CAD build for the part. Positions are in the model's coordinates, mm. Face numbers are marked on the shaded views. A direction names the side the tool comes from. Coordinates: 2 decimals unless noted, no trailing zeros. Write each loop counter-clockwise with the first axis right and the second up, starting at its lowest first coordinate (ties: lowest second). Pieces come first, ordered by that corner, then holes. Notation, with made-up numbers: (49.5, -2.75) - (59.5, -2.75) arc R23 ccw to (59.5, 30.25) - close; hole circle Ø11 at (20.5, 50). An arc over 180 degrees is marked (long way). Answer in a Markdown table with one row per item. Add a question column.
Q1. Band-saw the part on A-A (z = 28.5). List the corners of the cut face in (x, y).
Q2. Drill centre lines: line 1 along X through (y, z) = (-24, 7); line 2 along X through (y, z) = (-14, 20); line 3 along Z through (x, y) = (-16, 27). Where is each one in solid material? Low to high. Write a range as from..to.
Q3. Band-saw the part on C-C (x = -31.5). List the corners of the cut face in (y, z), and give its area (3 significant figures).
Q4. Band-saw the part on B-B (y = -18). List the corners of the cut face in (x, z).
Q5. Two-plate mould, pull along X, no slides. Class the marked faces 4, 5 and 6: +X half, -X half, draft (parallel to the pull), parting line (faces both ways), or undercut.
Q6. Pin check, flat tips, straight feed: pin 1 (4 mm diameter, centred on y = 12, z = 5.5, fed in from -X); pin 2 (10 mm diameter, centred on y = -17, z = 10, fed in from -X); pin 3 (1.5 mm diameter, centred on x = 15, y = 28.5, fed in from -Z). Stop position of each tip, or through.
Q7. 3-axis set-ups, long thin cutter, end or side, ignore diameter. For the marked faces 1, 2 and 3: which of +Z, -Z, +X, -X, +Y, -Y reach the whole face in a straight line?
```python
from build123d import *

# Parameters (mm, degrees)
F1_DEPTH     = 30
F3_DEPTH     = 30
F4_DEPTH     = 25
F5_T1_DEPTH  = 97.9548533656
F5_T3_DEPTH  = 20
F5_T5_DEPTH  = 20.7033743208
F5_T7_DEPTH  = 97.9794901198
F5_T9_DEPTH  = 20
F5_T12_ANGLE = 75.8911885194
F5_T14_ANGLE = 104.1088114806
F5_T16_ANGLE = 75.2928746344
F5_T20_DEPTH = 43.6443917162
F5_T23_ANGLE = 75.8339831116
F5_T25_ANGLE = 104.1660168884
F5_T27_ANGLE = 78.1908320725
F5_T31_DEPTH = 42.9024259572
F5_T37_DEPTH = 42.9024259572
F5_T41_DEPTH = 43.6443917162


# Not quite as in the source:
# - a fillet or chamfer that OpenCascade refuses, or shapes differently, is made with other operations: its cross-section is extruded or revolved along the edge and cut away or added
# - the program builds the solid bodies; features that only make, move or delete a surface that nothing else refers to are left out


with BuildPart() as f1:
    # F0 (on Top) → F1 (new body)
    with BuildSketch(Plane.XY):
        with BuildLine():
            Line((9.3227045948, 64.7266464915), (-11.3806697261, 64.7266464915))
            ThreePointArc((-11.3806697261, 64.7266464915), (-15.9925167381, 63.1411090315), (-18.6544287642, 59.0548777281))
            Line((-18.6544287642, 59.0548777281), (-42.5323117917, -35.9451222719))
            ThreePointArc((-42.5323117917, -35.9451222719), (-41.1730152936, -42.3852005206), (-35.2585527536, -45.2733535085))
            Line((-35.2585527536, -45.2733535085), (-15.2585527536, -45.2733535085))
            ThreePointArc((-15.2585527536, -45.2733535085), (-10.6776494918, -43.7118150354), (-8.004281346, -39.6774402567))
            Line((-8.004281346, -39.6774402567), (-0.1883919579, -9.9001294455))
            Line((-0.1883919579, -9.9001294455), (5.9601953638, -39.3082485958))
            ThreePointArc((5.9601953638, -39.3082485958), (8.571852392, -43.5940799733), (13.3014552741, -45.2733535085))
            Line((13.3014552741, -45.2733535085), (33.3014552741, -45.2733535085))
            ThreePointArc((33.3014552741, -45.2733535085), (39.2182193635, -42.3822473792), (40.5733853395, -35.9378608981))
            Line((40.5733853395, -35.9378608981), (16.5946346602, 59.0621391019))
            ThreePointArc((16.5946346602, 59.0621391019), (13.9315984654, 63.1434105808), (9.3227045948, 64.7266464915))
        make_face()
        with BuildLine():
            ThreePointArc((9.3227045948, 59.7266464915), (10.8590025517, 59.1989011879), (11.7466812833, 57.8384773616))
            Line((11.7466812833, 57.8384773616), (35.7254319626, -37.1615226384))
            ThreePointArc((35.7254319626, -37.1615226384), (35.2737099706, -39.3096514654), (33.3014552741, -40.2733535085))
            Line((33.3014552741, -40.2733535085), (13.3014552741, -40.2733535085))
            ThreePointArc((13.3014552741, -40.2733535085), (11.72492098, -39.7135956635), (10.8543686373, -38.2849852043))
            Line((10.8543686373, -38.2849852043), (3.2176150905, -1.7591059289))
            ThreePointArc((3.2176150905, -1.7591059289), (2.3470627478, -0.3304954698), (0.7705284538, 0.2292623753))
            Line((0.7705284538, 0.2292623753), (-0.7705284538, 0.2292623753))
            ThreePointArc((-0.7705284538, 0.2292623753), (-2.2974962077, -0.2912504491), (-3.188618923, -1.6360420419))
            Line((-3.188618923, -1.6360420419), (-12.8404622844, -38.4080490913))
            ThreePointArc((-12.8404622844, -38.4080490913), (-13.7315849996, -39.7528406842), (-15.2585527536, -40.2733535085))
            Line((-15.2585527536, -40.2733535085), (-35.2585527536, -40.2733535085))
            ThreePointArc((-35.2585527536, -40.2733535085), (-37.2300402669, -39.3106358459), (-37.6831390996, -37.1639430963))
            Line((-37.6831390996, -37.1639430963), (-13.8052560721, 57.8360569037))
            ThreePointArc((-13.8052560721, 57.8360569037), (-12.9179520634, 59.1981340048), (-11.3806697261, 59.7266464915))
            Line((-11.3806697261, 59.7266464915), (9.3227045948, 59.7266464915))
        make_face(mode=Mode.SUBTRACT)
    extrude(amount=F1_DEPTH)

    # F0 (on Top) → F3 (join)
    with BuildSketch(Plane.XY):
        with BuildLine():
            Line((35.7254319626, -37.1615226384), (11.7466812833, 57.8384773616))
            ThreePointArc((11.7466812833, 57.8384773616), (10.8590025517, 59.1989011879), (9.3227045948, 59.7266464915))
            Line((9.3227045948, 59.7266464915), (-11.3806697261, 59.7266464915))
            ThreePointArc((-11.3806697261, 59.7266464915), (-12.9179520634, 59.1981340048), (-13.8052560721, 57.8360569037))
            Line((-13.8052560721, 57.8360569037), (-37.6831390996, -37.1639430963))
            ThreePointArc((-37.6831390996, -37.1639430963), (-37.2300402669, -39.3106358459), (-35.2585527536, -40.2733535085))
            Line((-35.2585527536, -40.2733535085), (-15.2585527536, -40.2733535085))
            ThreePointArc((-15.2585527536, -40.2733535085), (-13.7315849996, -39.7528406842), (-12.8404622844, -38.4080490913))
            Line((-12.8404622844, -38.4080490913), (-3.188618923, -1.6360420419))
            ThreePointArc((-3.188618923, -1.6360420419), (-2.2974962077, -0.2912504491), (-0.7705284538, 0.2292623753))
            Line((-0.7705284538, 0.2292623753), (0.7705284538, 0.2292623753))
            ThreePointArc((0.7705284538, 0.2292623753), (2.3470627478, -0.3304954698), (3.2176150905, -1.7591059289))
            Line((3.2176150905, -1.7591059289), (10.8543686373, -38.2849852043))
            ThreePointArc((10.8543686373, -38.2849852043), (11.72492098, -39.7135956635), (13.3014552741, -40.2733535085))
            Line((13.3014552741, -40.2733535085), (33.3014552741, -40.2733535085))
            ThreePointArc((33.3014552741, -40.2733535085), (35.2737099706, -39.3096514654), (35.7254319626, -37.1615226384))
        make_face()
        Polygon((2.9763113208, 15.0989185788), (-2.9763113208, 15.0989185788), (-0.655874512, 25.3615314645), (0.655874512, 25.3615314645), align=None, mode=Mode.SUBTRACT)
    extrude(amount=F3_DEPTH)

    # F0 (on Top) → F4 (cut)
    with BuildSketch(Plane.XY):
        with BuildLine():
            Line((35.7254319626, -37.1615226384), (11.7466812833, 57.8384773616))
            ThreePointArc((11.7466812833, 57.8384773616), (10.8590025517, 59.1989011879), (9.3227045948, 59.7266464915))
            Line((9.3227045948, 59.7266464915), (-11.3806697261, 59.7266464915))
            ThreePointArc((-11.3806697261, 59.7266464915), (-12.9179520634, 59.1981340048), (-13.8052560721, 57.8360569037))
            Line((-13.8052560721, 57.8360569037), (-37.6831390996, -37.1639430963))
            ThreePointArc((-37.6831390996, -37.1639430963), (-37.2300402669, -39.3106358459), (-35.2585527536, -40.2733535085))
            Line((-35.2585527536, -40.2733535085), (-15.2585527536, -40.2733535085))
            ThreePointArc((-15.2585527536, -40.2733535085), (-13.7315849996, -39.7528406842), (-12.8404622844, -38.4080490913))
            Line((-12.8404622844, -38.4080490913), (-3.188618923, -1.6360420419))
            ThreePointArc((-3.188618923, -1.6360420419), (-2.2974962077, -0.2912504491), (-0.7705284538, 0.2292623753))
            Line((-0.7705284538, 0.2292623753), (0.7705284538, 0.2292623753))
            ThreePointArc((0.7705284538, 0.2292623753), (2.3470627478, -0.3304954698), (3.2176150905, -1.7591059289))
            Line((3.2176150905, -1.7591059289), (10.8543686373, -38.2849852043))
            ThreePointArc((10.8543686373, -38.2849852043), (11.72492098, -39.7135956635), (13.3014552741, -40.2733535085))
            Line((13.3014552741, -40.2733535085), (33.3014552741, -40.2733535085))
            ThreePointArc((33.3014552741, -40.2733535085), (35.2737099706, -39.3096514654), (35.7254319626, -37.1615226384))
        make_face()
        Polygon((2.9763113208, 15.0989185788), (-2.9763113208, 15.0989185788), (-0.655874512, 25.3615314645), (0.655874512, 25.3615314645), align=None, mode=Mode.SUBTRACT)
    extrude(amount=F4_DEPTH, mode=Mode.SUBTRACT)

    # F5: chamfer of 5 on 1 edges, made by hand

    # F5_s2 → F5_t1 (cut)
    with BuildSketch(Plane(origin=(12.8527529512, 51.135669312, 0), x_dir=(0, 0, 1), z_dir=(-0.2437641649, -0.9698345384, 0))):
        Polygon((0, 27.4871722621), (5, 32.4871722621), (0, 32.4871722621), align=None)
    extrude(amount=F5_T1_DEPTH, mode=Mode.SUBTRACT)

    # F5_s4 → F5_t3 (cut)
    with BuildSketch(Plane.YZ.offset(-35.2585527536)):
        Polygon((-40.2733535085, 0), (-45.2733535085, 5), (-45.2733535085, 0), align=None)
    extrude(amount=F5_T3_DEPTH, mode=Mode.SUBTRACT)

    # F5_s6 → F5_t5 (cut)
    with BuildSketch(Plane.YZ.offset(-11.3806697261)):
        Polygon((64.7266464915, 5), (59.7266464915, 0), (64.7266464915, 0), align=None)
    extrude(amount=F5_T5_DEPTH, mode=Mode.SUBTRACT)

    # F5_s8 → F5_t7 (cut)
    with BuildSketch(Plane(origin=(10.9578014799, -43.4130682832, 0), x_dir=(0, 0, 1), z_dir=(-0.2447323481, 0.9695906754, 0))):
        Polygon((5, 30.5444190123), (0, 25.5444190123), (0, 30.5444190123), align=None)
    extrude(amount=F5_T7_DEPTH, mode=Mode.SUBTRACT)

    # F5_s10 → F5_t9 (cut)
    with BuildSketch(Plane.YZ.offset(13.3014552741)):
        Polygon((-40.2733535085, 0), (-45.2733535085, 5), (-45.2733535085, 0), align=None)
    extrude(amount=F5_T9_DEPTH, mode=Mode.SUBTRACT)

    # F5_s11 → F5_t12 (revolve, cut)
    with BuildSketch(Plane.YZ.offset(-11.3806697261)):
        Polygon((59.7266464915, 0), (64.7266464915, 5), (64.7266464915, 0), align=None)
    revolve(axis=Axis((-11.3806697261, 57.2266464915, 0), (0, 0, 1)), revolution_arc=F5_T12_ANGLE, mode=Mode.SUBTRACT)

    # F5_s13 → F5_t14 (revolve, cut)
    with BuildSketch(Plane(origin=(-11.0251300763, -43.864330688, 0), x_dir=(0, 0, 1), z_dir=(0.2437641649, 0.9698345384, 0))):
        Polygon((0, -27.4871722621), (5, -32.4871722621), (0, -32.4871722621), align=None)
    revolve(axis=Axis((-35.2585527536, -37.7733535085, 0), (0, 0, 1)), revolution_arc=F5_T14_ANGLE, mode=Mode.SUBTRACT)

    # F5_s15 → F5_t16 (revolve, cut)
    with BuildSketch(Plane.YZ.offset(-15.2585527536)):
        Polygon((-40.2733535085, 0), (-45.2733535085, 5), (-45.2733535085, 0), align=None)
    revolve(axis=Axis((-15.2585527536, -37.7733535085, 0), (0, 0, 1)), revolution_arc=F5_T16_ANGLE, mode=Mode.SUBTRACT)


with BuildPart() as f5_tool18:
    # F5_s19 → F5_t20 (new body)
    with BuildSketch(Plane(origin=(-10.2591099413, -39.0855973263, 0), x_dir=(0, 0, 1), z_dir=(0.2538782331, 0.9672361877, 0))):
        Polygon((0, -2.6687921481), (5, 2.3312078519), (0, 2.3312078519), align=None)
    extrude(amount=F5_T20_DEPTH)

    split(bisect_by=Plane(origin=(-2.1637067448, -0.4523832276, 0), x_dir=(0, 0, 1), z_dir=(-0.9788346547, -0.2046526783, 0)), keep=Keep.TOP)


with BuildPart() as f1_1:
    add(f1.part)

    # F5_t17: cut F5_tool18
    add(f5_tool18.part, mode=Mode.SUBTRACT)

    # F5_s22 → F5_t23 (revolve, cut)
    with BuildSketch(Plane(origin=(-13.0209491994, 51.5869317168, 0), x_dir=(0, 0, 1), z_dir=(0.2447323481, -0.9695906754, 0))):
        Polygon((5, -30.5444190123), (0, -25.5444190123), (0, -30.5444190123), align=None)
    revolve(axis=Axis((9.3227045948, 57.2266464915, 0), (0, 0, 1)), revolution_arc=F5_T23_ANGLE, mode=Mode.SUBTRACT)

    # F5_s24 → F5_t25 (revolve, cut)
    with BuildSketch(Plane.YZ.offset(33.3014552741)):
        Polygon((-40.2733535085, 0), (-45.2733535085, 5), (-45.2733535085, 0), align=None)
    revolve(axis=Axis((33.3014552741, -37.7733535085, 0), (0, 0, 1)), revolution_arc=F5_T25_ANGLE, mode=Mode.SUBTRACT)

    # F5_s26 → F5_t27 (revolve, cut)
    with BuildSketch(Plane(origin=(8.1239021086, -38.8558653682, 0), x_dir=(0, 0, 1), z_dir=(-0.2046526783, 0.9788346547, 0))):
        Polygon((0, 2.7895074164), (5, -2.2104925836), (0, -2.2104925836), align=None)
    revolve(axis=Axis((13.3014552741, -37.7733535085, 0), (0, 0, 1)), revolution_arc=F5_T27_ANGLE, mode=Mode.SUBTRACT)


with BuildPart() as f5_tool29:
    # F5_s30 → F5_t31 (new body)
    with BuildSketch(Plane(origin=(-0.6561942692, 3.1385159299, 0), x_dir=(0, 0, 1), z_dir=(0.2046526783, -0.9788346547, 0))):
        Polygon((0, -2.7895074164), (5, 2.2104925836), (0, 2.2104925836), align=None)
    extrude(amount=F5_T31_DEPTH)

    split(bisect_by=Plane(origin=(2.2548285953, -0.5918429304, 0), x_dir=(0, 0, 1), z_dir=(0.9672361877, -0.2538782331, 0)), keep=Keep.TOP)


with BuildPart() as f1_2:
    add(f1_1.part)

    # F5_t28: cut F5_tool29
    add(f5_tool29.part, mode=Mode.SUBTRACT)


with BuildPart() as f5_tool35:
    # F5_s36 → F5_t37 (new body)
    with BuildSketch(Plane(origin=(-0.6561942692, 3.1385159299, 0), x_dir=(0, 0, 1), z_dir=(0.2046526783, -0.9788346547, 0))):
        Polygon((0, -2.7895074164), (5, 2.2104925836), (0, 2.2104925836), align=None)
    extrude(amount=F5_T37_DEPTH)

    split(bisect_by=Plane(origin=(2.2548285953, -0.5918429304, 0), x_dir=(0, 0, 1), z_dir=(-0.9672361877, 0.2538782331, 0)), keep=Keep.TOP)


with BuildPart() as f5_tool39:
    # F5_s40 → F5_t41 (new body)
    with BuildSketch(Plane(origin=(-10.2591099413, -39.0855973263, 0), x_dir=(0, 0, 1), z_dir=(0.2538782331, 0.9672361877, 0))):
        Polygon((0, -2.6687921481), (5, 2.3312078519), (0, 2.3312078519), align=None)
    extrude(amount=F5_T41_DEPTH)

    split(bisect_by=Plane(origin=(-2.1637067448, -0.4523832276, 0), x_dir=(0, 0, 1), z_dir=(0.9788346547, 0.2046526783, 0)), keep=Keep.TOP)


with BuildPart() as f5_tool35_1:
    add(f5_tool35.part)

    # F5_t43: intersect F5_tool39
    add(f5_tool39.part, mode=Mode.INTERSECT)


with BuildPart() as f1_3:
    add(f1_2.part)

    # F5_t33: cut F5_tool35
    add(f5_tool35_1.part, mode=Mode.SUBTRACT)


solid = f1_3.part
```
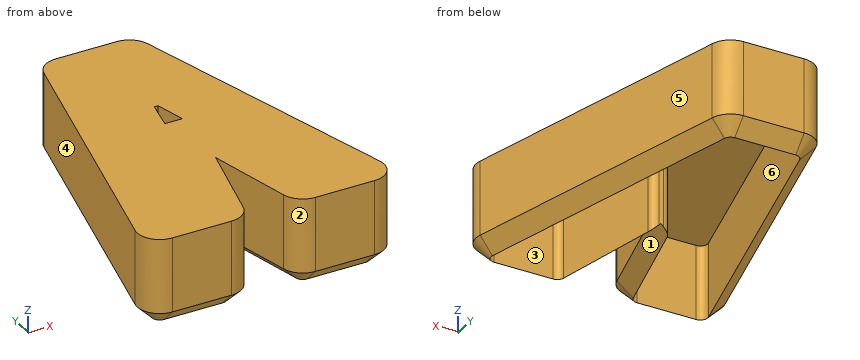
Checked values:
| question | item | result |
|---|---|---|
| 1 | outline | (-42.53, -35.95) arc R7.5 ccw to (-35.26, -45.27) - (-15.26, -45.27) arc R7.5 ccw to (-8, -39.68) - (-0.19, -9.9) - (5.96, -39.31) arc R7.5 ccw to (13.3, -45.27) - (33.3, -45.27) arc R7.5 ccw to (40.57, -35.94) - (16.59, 59.06) arc R7.5 ccw to (9.32, 64.73) - (-11.38, 64.73) arc R7.5 ccw to (-18.65, 59.05) - close; hole (-2.98, 15.1) - (2.98, 15.1) - (0.66, 25.36) - (-0.66, 25.36) - close |
| 2 | line 1 | x = -39.53..-34.37, -9.06..-3.89, 2.76..7.87, 32.4..37.56 |
| 2 | line 2 | x = -37.02..-31.86, -6.43..-1.26, 0.67..5.78, 29.88..35.04 |
| 2 | line 3 | z = 25..30 |
| 3 | outline | (-45.27, 5) - (-40.27, 0) - (-40.27, 25) - (-12.56, 25) - (-12.56, 0) - (7.95, 5) - (7.95, 30) - (-45.27, 30) - close |
| 3 | area | 840 mm² |
| 4 | outline | (-38.02, 5) - (-32.87, 0) - (-32.87, 25) - (-7.48, 25) - (-7.48, 0) - (-2.31, 5) - (-2.31, 30) - (-38.02, 30) - close; (1.51, 5) - (6.61, 0) - (6.61, 25) - (30.89, 25) - (30.89, 0) - (36.05, 5) - (36.05, 30) - (1.51, 30) - close |
| 5 | face 4 | -X half |
| 5 | face 5 | +X half |
| 5 | face 6 | undercut |
| 6 | pin 1 | stops at x = -30.98 |
| 6 | pin 2 | stops at x = -39.03 |
| 6 | pin 3 | stops at z = 25 |
| 7 | face 1 | -Z, -Y |
| 7 | face 2 | +Z, -Z, -Y |
| 7 | face 3 | -Z |
